Input: part model. Units: mm. Frame: model coordinates. Face numbers are marked on the shaded views. A direction names the side the tool comes from. Coordinates: 2 decimals unless noted, no trailing zeros. Write each loop counter-clockwise with the first axis right and the second up, starting at its lowest first coordinate (ties: lowest second). Pieces come first, ordered by that corner, then holes. Notation, with made-up numbers: M 35,83.5 L 61,83.5 A17 cw 61,102.5 Z; hole C 68,50 d11. An arc over 180 degrees is marked long. Write each question's results on one line, items separated by ' | '. Start each with the question number.
1. Set-up query: the marked faces 1, 2 and 3. Return all of +Z, -Z, +X, -X, +Y, -Y with unobstructed straight access to the full face (end or side cutting, diameter ignored); none if empty.
2. Section query B-B, the plane y = 16.5. Output: boundary loops of the cut face in (x, z).
3. Ray query, probe 1 along Z at (x, y) = (6.8, 26.2); probe 2 along X at (y, z) = (4, 7.75); probe 3 along Y at (x, z) = (7.6, 0). Return the intervals inside material, ascending.
4. Section query D-D, the plane y = 29.5. Output: boundary loops of the cut face in (x, z), and give its area (3 significant figures).
5. Section query C-C, the plane z = 1.25. Output: boundary loops of the cut face in (x, y), and give its area (3 significant figures).
6. Section query A-A, the plane z = 6.25. Output: boundary loops of the cut face in (x, y).
7. Pull-direction query (X, two-part tool) for the marked faces 4, 5 and 6; classes: +X half, -X half, draft (parallel to the pull), parting line (faces both ways), or undercut.
8. First-contact query: pin 1 (8 mm diameter, centred on y = 5, z = -0.5, fed in from -X); pin 2 (2.5 mm diameter, centred on x = 11, y = 1.5, fed in from +Z); pin 3 (7 mm diameter, centred on y = 25.5, z = -1.5, fed in from +X); pin 4 (4 mm diameter, centred on x = -12.5, z = -4, fed in from +Y). Flat tips, straight axial feed; report the tip coordinate or a pass-through.
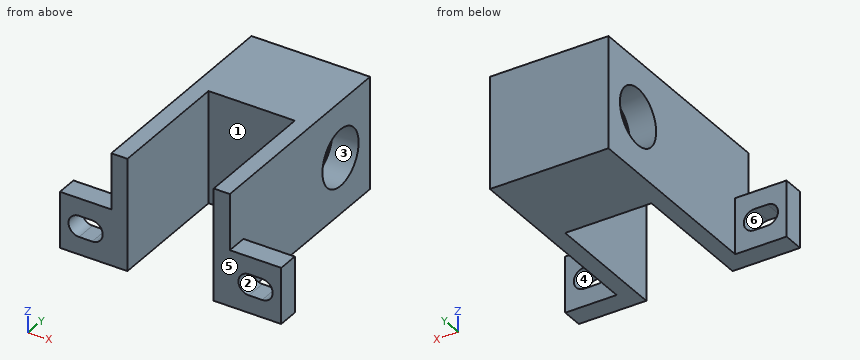
Autodesk Inventor part; units mm, degrees
ref_plane "YZ Plane" through (0, 0, 0) normal (1, 0, 0) x (0, 1, 0)
ref_plane "XZ Plane" through (0, 0, 0) normal (0, 1, 0) x (-1, 0, 0)
ref_plane "XY Plane" through (0, 0, 0) normal (0, 0, 1) x (1, 0, 0)
sketch "Sketch1" plane through (0, 0, 0) normal (0, 1, 0) x (-1, 0, 0)
  line L0 (-9, 8.5) -> (9, 8.5)
  line L1 (9, 8.5) -> (9, -8.5)
  line L2 (9, -8.5) -> (-9, -8.5)
  line L3 (-9, -8.5) -> (-9, 8.5)
  line L4 (-9, 8.5) -> (9, -8.5) construction
  line L5 (9, 8.5) -> (-9, -8.5) construction
  point P0 (0, 0)
  dimension "d0" = 18
  dimension "d1" = 17
extrude "Extrusion1" add sketch "Sketch1" along normal blind 33.2
sketch "Sketch2" plane through (0, 0, 0) normal (0, -1, 0) x (1, 0, 0)
  line L0 (9, -8.5) -> (-9, -8.5)
  line L1 (-6.55, 8.5) -> (6.55, 8.5)
  line L2 (6.55, 8.5) -> (6.55, -8.5)
  line L3 (6.55, -8.5) -> (-6.55, -8.5)
  line L4 (-6.55, -8.5) -> (-6.55, 8.5)
  line L5 (-6.55, 8.5) -> (6.55, -8.5) construction
  line L6 (6.55, 8.5) -> (-6.55, -8.5) construction
  point P0 (0, 0)
  point P1 (-6.55, -8.5)
  dimension "d4" = 13.1
extrude "Extrusion2" cut sketch "Sketch2" against normal blind 19.2
sketch "Sketch4" plane through (0, 0, 0) normal (0, -1, 0) x (1, 0, 0)
  line L0 (9, 8.5) -> (9, -8.5)
  line L1 (9, 0) -> (16.8, 0)
  line L2 (16.8, 0) -> (16.8, -8.5)
  line L3 (16.8, -8.5) -> (9, -8.5)
  line L4 (9, -8.5) -> (9, 0)
  line L5 (-9, -8.5) -> (-9, 8.5)
  line L6 (-9, -8.5) -> (-16.8, -8.5)
  line L7 (-16.8, -8.5) -> (-16.8, 0)
  line L8 (-16.8, 0) -> (-9, 0)
  line L9 (-9, 0) -> (-9, -8.5)
  point P0 (0, 0)
  dimension "d7" = 7.8
  dimension "d8" = 7.8
extrude "Extrusion3" add sketch "Sketch4" against normal blind 3.2
sketch "Sketch5" plane through (0, 3.2, 0) normal (0, 1, 0) x (1, 0, 0)
  line L0 (9, 0) -> (9, 8.5) construction
  line L1 (9, 4.25) -> (11.9, 4.25) construction
  circle A0 centre (11.9, 4.25) radius 1.6
  line L2 (11.9, 4.25) -> (13.9, 4.25) construction
  circle A1 centre (13.9, 4.25) radius 1.6
  line L3 (13.9, 5.85) -> (11.9, 5.85)
  line L4 (11.9, 2.65) -> (13.9, 2.65)
  line L5 (-9, 8.5) -> (-9, 0) construction
  line L6 (-9, 4.25) -> (-11.9, 4.25) construction
  line L7 (-11.9, 4.25) -> (-13.9, 4.25) construction
  circle A2 centre (-11.9, 4.25) radius 1.6
  circle A3 centre (-13.9, 4.25) radius 1.6
  line L8 (-13.9, 5.85) -> (-11.9, 5.85)
  line L9 (-13.9, 2.65) -> (-11.9, 2.65)
  point P0 (0, 0)
  dimension "d11" = 2.9
  dimension "d12" = 3.2
  dimension "d13" = 2
  dimension "d14" = 3.2
  dimension "d17" = 2.9
  dimension "d18" = 2
  dimension "d19" = 3.2
  dimension "d20" = 3.2
extrude "Extrusion4" cut sketch "Sketch5" against normal through all
sketch "Sketch6" plane through (9, 0, 8.5) normal (1, 0, 0) x (0, 0, -1)
  line L0 (0, 33.2) -> (17, 33.2) construction
  line L1 (8.5, 33.2) -> (8.5, 26.2) construction
  circle A0 centre (8.5, 26.2) radius 4
  point P0 (8.5, 0)
  dimension "d21" = 7
  dimension "d22" = 8
extrude "Extrusion5" cut sketch "Sketch6" against normal through all
sketch "Sketch8" plane through (9, 0, 8.5) normal (1, 0, 0) x (0, 0, -1)
  line L0 (0, 33.2) -> (17, 33.2) construction
  line L1 (8.5, 33.2) -> (8.5, 26.2) construction
  point P0 (8.5, 0)
  dimension "d33" = 7
hole "Hole2" at (9, 26.2, 0) direction (-1, 0, 0) diameter 8.566 depth 4
sketch "Sketch9" plane through (-9, 0, 8.5) normal (-1, 0, 0) x (0, 0, 1)
  line L0 (-17, 33.2) -> (0, 33.2) construction
  line L1 (-8.5, 33.2) -> (-8.5, 26.2) construction
  point P0 (-8.5, 0)
  dimension "d41" = 7
hole "Hole3" at (-9, 26.2, 0) direction (1, 0, 0) diameter 8.566 depth 4
properties part number "ADAPTER_AOM-brimrose-watercooled-cover"
Answer:
1) face 1: +Z, -Z, -Y | face 2: +Y, -Y | face 3: +X
2) outline: M -9,-8.5 L -6.55,-8.5 L -6.55,8.5 L -9,8.5 Z; M 6.55,-8.5 L 9,-8.5 L 9,8.5 L 6.55,8.5 Z
3) probe 1: -8.5 to -4.28, 4.28 to 8.5 | probe 2: -9 to -6.55, 6.55 to 9 | probe 3: 0 to 21.92, 30.48 to 33.2
4) outline: M -9,-8.5 L 9,-8.5 L 9,-2.73 L 5,-2.73 L 5,-2.26 L -5,-2.26 L -5,-2.73 L -9,-2.73 Z; M -9,2.73 L -5,2.73 L -5,2.26 L 5,2.26 L 5,2.73 L 9,2.73 L 9,8.5 L -9,8.5 Z | area: 217 mm^2
5) outline: M -9,0 L -6.55,0 L -6.55,19.2 L 6.55,19.2 L 6.55,0 L 9,0 L 9,22.1 L 5,22.1 L 5,22.4 L -5,22.4 L -5,22.1 L -9,22.1 Z; M -9,30.3 L -5,30.3 L -5,30 L 5,30 L 5,30.3 L 9,30.3 L 9,33.2 L -9,33.2 Z | area: 205 mm^2
6) outline: M -9,0 L -6.55,0 L -6.55,19.2 L 6.55,19.2 L 6.55,0 L 9,0 L 9,33.2 L -9,33.2 Z
7) face 4: undercut | face 5: draft | face 6: undercut
8) pin 1: x = -16.8 | pin 2: z = 0 | pin 3: x = 9 | pin 4: y = 3.2
